Part model, mm, in its own coordinate system. A direction names the side the tool comes from. Give positions to 0.01 mm unless a question says otherwise; leave off trailing zeros. Loops run counter-clockwise (first coordinate to the right, second up) from the corner with the lowest first, then second, coordinate; pieces in that order, holes last. Notation, with made-up numbers: (63, -25) -> (93, -25) arc R29 ccw to (93, 3) -> close; hole circle Ø6 at (75, 53). An arc over 180 degrees is marked (long way). One line per question, with ' | ' between items.
```python
from build123d import *

# Parameters (mm, degrees)
SKETCH1_R           = 9.5
BOSS_EXTRUDE1_DEPTH = 25
SKETCH2_R           = 4
CUT_EXTRUDE1_DEPTH  = 10
SKETCH3_R           = 2.5
CUT_EXTRUDE2_DEPTH  = 10


with BuildPart() as part:
    # Sketch1 → Boss-Extrude1 (new body)
    with BuildSketch(Plane.XY):
        Circle(SKETCH1_R)
    extrude(amount=BOSS_EXTRUDE1_DEPTH)

    # Sketch2 → Cut-Extrude1 (cut)
    with BuildSketch(Plane.XY.offset(25)):
        Circle(SKETCH2_R)
    extrude(amount=-CUT_EXTRUDE1_DEPTH, mode=Mode.SUBTRACT)

    # Sketch3 → Cut-Extrude2 (cut)
    with BuildSketch(Plane(origin=(0, 0, 0), x_dir=(-1, 0, 0), z_dir=(0, 0, -1))):
        Circle(SKETCH3_R)
    extrude(amount=-CUT_EXTRUDE2_DEPTH, mode=Mode.SUBTRACT)


solid = part.part
```
1) Saw through at A-A (y = 0). Give the cut face in (x, z), and give its area (3 significant figures).
Found:
outline: (-9.5, 0) -> (-2.5, 0) -> (-2.5, 10) -> (2.5, 10) -> (2.5, 0) -> (9.5, 0) -> (9.5, 25) -> (4, 25) -> (4, 15) -> (-4, 15) -> (-4, 25) -> (-9.5, 25) -> close | area: 345 mm2
2) Pin check, flat tips, straight feed: P1, Ø1.5, axis at x = -7.5, z = 12.5, coming from the +Y side; P2, Ø8, axis at x = 7, z = 16.5, coming from the +Y side; P3, Ø4, axis at x = 4.5, z = 21.5, coming from the +Y side. Stop position of each tip, or through.
Found:
P1: y = 6.68 | P2: y = 9.01 | P3: y = 9.17
3) Saw through at D-D (x = -3.5). Give the cut face in (y, z), and give its area (3 significant figures).
Found:
outline: (-8.83, 0) -> (8.83, 0) -> (8.83, 25) -> (1.94, 25) -> (1.94, 15) -> (-1.94, 15) -> (-1.94, 25) -> (-8.83, 25) -> close | area: 403 mm2
4) Tool access for faces 1 (the flat face through (0, 0, 15)), 2 (the flat face through (2, -2, 0)), 3 (the cylindrical face through (0.54, -2.44, 4.93)): list every direction of +Z, -Z, +X, -X, +Y, -Y with a clear straight run to the whole face (end or side of a thin tool).
Found:
face 1: +Z | face 2: -Z, +X, -X, +Y, -Y | face 3: -Z
5) Drill centre lines: line 1 (Y direction, x = 0, z = 18); line 2 (Y direction, x = 0, z = 7.75); line 3 (Z direction, x = -0.25, y = 2.25). Where is each one in solid material? Low to high.
Found:
line 1: -9.5 to -4, 4 to 9.5 | line 2: -9.5 to -2.5, 2.5 to 9.5 | line 3: 10 to 15
6) Saw through at B-B (z = 4.75). Give the cut face in (x, y), and give its area (3 significant figures).
Found:
outline: circle Ø19 at (0, 0); hole circle Ø5 at (0, 0) | area: 264 mm2
7) Pull direction Y, two halves, no side cores. Call faces 4 (the cylindrical face through (-0.867, -3.905, 20.07)), 5 (the cylindrical face through (4.38, -8.43, 12.32)), 6 (the flat face through (4, -2, 25)): pulls with the +Y half, pulls with the -Y half, needs draft (parallel to the pull), parting line crosses it, or undercut.
Found:
face 4: undercut | face 5: parting line crosses it | face 6: needs draft
